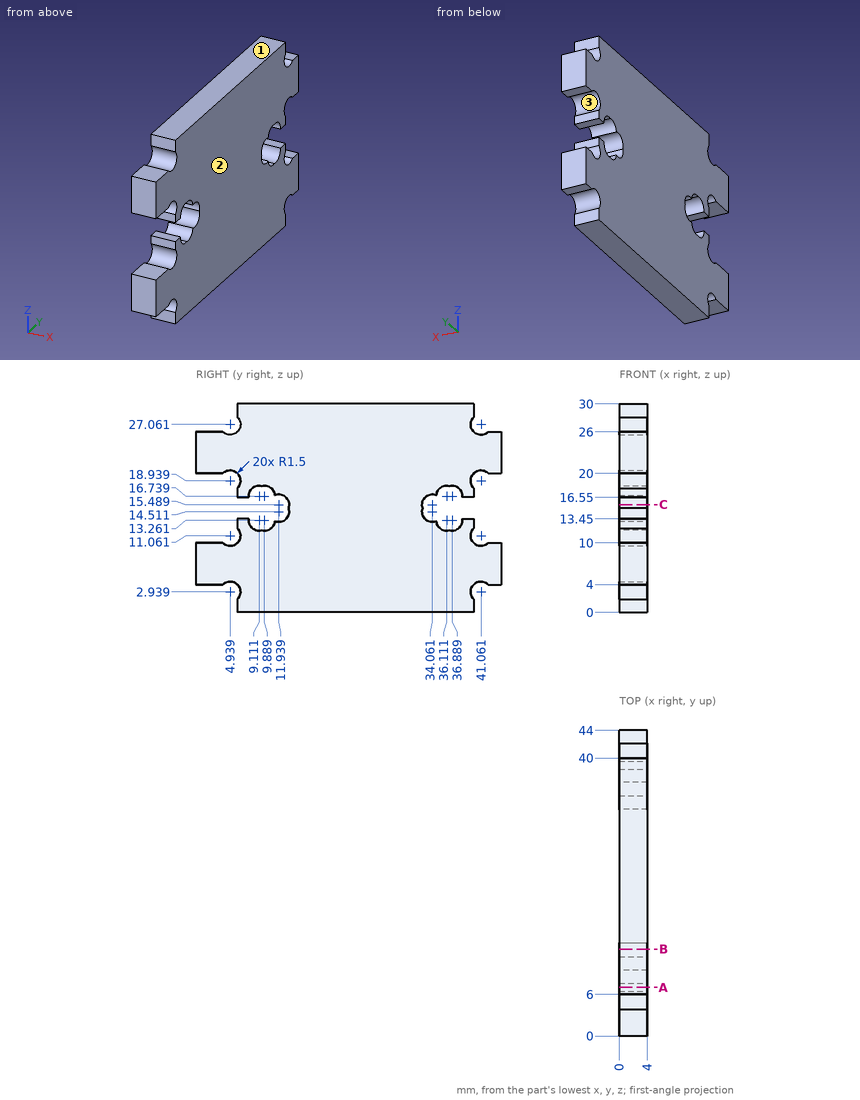
Input: dimensioned drawing with shaded views. Units: mm. Origin: part minimum x, y, z. Coordinates: 2 decimals unless noted, no trailing zeros. Order: outer loops, then holes, each group sorted by start corner. A loop starts at its lowest first (then second) coordinate and runs counter-clockwise, first axis right, second up. Notation, with made-up numbers: M -24.5,-18.75 L 12.5,-18.75 A21 cw 12.5,-1.75 Z; hole C 61.25,70 d3. An arc over 180 degrees is marked long. Write each question's results on one line, items separated by ' | '. Start each with the question number.
Item 1: Cut plane B-B (y = 12.5). Return loops of the section in (x, z).
Item 2: Draft query along Z for the marked faces 1, 2 and 3. Return one class per face: pulls with the +Z half, pulls with the -Z half, needs draft (parallel to the pull), parting line crosses it, or undercut.
Item 3: First-contact query: pin 1 Ø2 at (x, y) = (3, 43) entering from +Z; pin 2 Ø1.5 at (x, z) = (1, 29) entering from +Y; pin 3 Ø1.5 at (x, y) = (2.5, 43.5) entering from -Z. Flat tips, straight axial feed; report the tip coordinate or a pass-through.
Item 4: Cut plane C-C (z = 15.5). Return loops of the section in (x, y), and give its area (3 significant figures).
Item 5: Cut plane A-A (y = 7). Return loops of the section in (x, z).
Item 6: Line query: probe 1 along Z at (x, y) = (1, 39); probe 2 along Z at (x, y) = (2.3, 5); probe 3 along Y at (x, z) = (2.6, 17.5). Output: solid intervals per line, ascending.
Checked values:
1) outline: M 0,0 L 4,0 L 4,13.12 L 0,13.12 Z; M 0,16.88 L 4,16.88 L 4,30 L 0,30 Z
2) face 1: pulls with the +Z half | face 2: needs draft | face 3: undercut
3) pin 1: stops at z = 26 | pin 2: stops at y = 40 | pin 3: stops at z = 4
4) outline: M 0,13.44 L 4,13.44 L 4,32.56 L 0,32.56 Z | area: 76.5 mm2
5) outline: M 0,0 L 4,0 L 4,13.45 L 0,13.45 Z; M 0,16.55 L 4,16.55 L 4,30 L 0,30 Z
6) probe 1: z = 0 to 13.45, 16.55 to 30 | probe 2: z = 4.44 to 9.56, 20.44 to 25.56 | probe 3: y = 6 to 7.82, 11.18 to 34.82, 38.18 to 40
